For this review, take the finished solid that the model builds, in its own axes (mm). A direction names the side the tool comes from. Coordinates: 2 decimals unless noted, no trailing zeros. Loops run counter-clockwise (first coordinate to the right, second up) from the corner with the lowest first, then second, coordinate; pieces in that order, holes last. Notation, with made-up numbers: (-7, 27.25) -> (48, 27.25) arc R30 cw to (48, 58.25) -> close; hole circle Ø9 at (-33.75, -1). An arc over 180 degrees is marked (long way). One line per item, written item: value.
from build123d import *

# Parameters (mm, degrees)
IZIM1_W                                        = 46
IZIM1_H                                        = 22
Y_KSEKLIK_EKSTR_ZYON1_DEPTH                    = 35
IZIM2_W                                        = 40
IZIM2_H                                        = 22
KES_EKSTR_ZYON1_DEPTH                          = 32
RADYUS1_R                                      = 11
PAH1_SIZE                                      = 3
IZIM3_W                                        = 5
IZIM3_H                                        = 10
KES_EKSTR_ZYON2_DEPTH                          = 20
FEDER5_REACH                                   = 46.833
IZIM8_WALL_W                                   = 96.666047784
IZIM8_WALL_H                                   = 6
AYNALAMA4_COPY_1_REACH                         = 46.833
AYNALAMA4_COPY_1_SKETCH_W                      = 96.666047784
AYNALAMA4_COPY_1_SKETCH_H                      = 6
IZIM10_R                                       = 3.1
KES_EKSTR_ZYON4_DEPTH                          = 59.838762733
IZIM12_R                                       = 3.1
Y_KSEKLIK_EKSTR_ZYON3_DEPTH                    = 3
M3_D_Z_BA_L_MAKINE_VIDAS_IN_HAV_A1_D           = 2.5
M3_D_Z_BA_L_MAKINE_VIDAS_IN_HAV_A1_CSINK_D     = 3.1
M3_D_Z_BA_L_MAKINE_VIDAS_IN_HAV_A1_CSINK_ANGLE = 90
IZIM18_R                                       = 4
Y_KSEKLIK_EKSTR_ZYON4_DEPTH                    = 62.22
IZIM19_W                                       = 4
IZIM19_H                                       = 4
KES_EKSTR_ZYON5_DEPTH                          = 10
RADYUS2_R                                      = 1
Y_KSEKLIK_EKSTR_ZYON5_DEPTH                    = 2
Y_KSEKLIK_EKSTR_ZYON5_DEPTH_BACK               = 2
IZIM21_W                                       = 6
IZIM21_H                                       = 6
IZIM22_R                                       = 1.5
KES_EKSTR_ZYON6_DEPTH                          = 9
IZIM23_R                                       = 2.251355404
KES_EKSTR_ZYON7_DEPTH                          = 2
RADYUS3_R                                      = 1
M2_D_Z_BA_L_MAKINE_VIDAS_IN_HAV_A2_D           = 2
M2_D_Z_BA_L_MAKINE_VIDAS_IN_HAV_A2_DEPTH       = 46
M2_D_Z_BA_L_MAKINE_VIDAS_IN_HAV_A2_CSINK_D     = 4.4
M2_D_Z_BA_L_MAKINE_VIDAS_IN_HAV_A2_CSINK_ANGLE = 90
M2_D_Z_BA_L_MAKINE_VIDAS_IN_HAV_A2_TIP         = 0.600860619


# Read off the part's stored shape, not the designer's step: M2 Düz Başlı Makine Vidası İçin Havşa1
with BuildPart() as part:
    # Çizim1 → Yükseklik-Ekstrüzyon1 (new body)
    with BuildSketch(Plane(origin=(0, 0, 0), x_dir=(0, 0, -1), z_dir=(1, 0, 0))):
        Rectangle(IZIM1_W, IZIM1_H)
    extrude(amount=Y_KSEKLIK_EKSTR_ZYON1_DEPTH)

    # Çizim2 → Kes-Ekstrüzyon1 (cut)
    with BuildSketch(Plane(origin=(35, 0, 0), x_dir=(0, 0, -1), z_dir=(1, 0, 0))):
        Rectangle(IZIM2_W, IZIM2_H)
    extrude(amount=-KES_EKSTR_ZYON1_DEPTH, mode=Mode.SUBTRACT)

    # Radyus1
    radyus1_edges = [part.edges().sort_by_distance(p)[0] for p in [
        (35, -11, 21.5),
        (35, 11, 21.5),
        (35, -11, -21.5),
        (35, 11, -21.5),
    ]]
    fillet(radyus1_edges, radius=RADYUS1_R - 0.0001)  # a hair under: the kernel refuses the full size

    # Pah1
    pah1_edges = [part.edges().sort_by_distance(p)[0] for p in [
        (0, 0, 23),
        (0, 0, -23),
    ]]
    chamfer(pah1_edges, length=PAH1_SIZE)

    # Çizim3 → Kes-Ekstrüzyon2 (cut)
    with BuildSketch(Plane(origin=(-10, 0, 10), x_dir=(0.7071067811865468, 0, 0.7071067811865483), z_dir=(-0.7071067811865483, 0, 0.7071067811865468))):
        with Locations((16.262135624, 0)):
            Rectangle(IZIM3_W, IZIM3_H)
    kes_ekstr_zyon2 = extrude(amount=-KES_EKSTR_ZYON2_DEPTH, mode=Mode.SUBTRACT)

    # M2 Düz Başlı Makine Vidası İçin Havşa1 ou → M2 Düz Başlı Makine Vidası İçin Havşa1 (revolve, cut)
    with BuildSketch(Plane(origin=(24, -8, 0), x_dir=(1, 0, 0), z_dir=(0, -1, 0))):
        Polygon((0, 20), (1, 20), (1, 22.7), (1.3, 23), (0, 23), align=None)
    m2_d_z_ba_l_makine_vidas_in_hav_a1 = revolve(axis=Axis((24, -8, 0), (0, 0, 1)), mode=Mode.SUBTRACT)

    # M2 D_z Ba_l_ Makine Vidas_ _in Hav_a 2 → M2 D_z Ba_l_ Makine Vidas_ _in Hav_a1 2 (revolve, cut)
    with BuildSketch(Plane(origin=(32, 0, 0), x_dir=(1, 0, 0), z_dir=(0, -1, 0))):
        Polygon((0, 20), (1, 20), (1, 22.7), (1.3, 23), (0, 23), align=None)
    m2_d_z_ba_l_makine_vidas_in_hav_a1_2 = revolve(axis=Axis((32, 0, 0), (0, 0, 1)), mode=Mode.SUBTRACT)

    # M2 D_z Ba_l_ Makine Vidas_ _in Hav_a 3 → M2 D_z Ba_l_ Makine Vidas_ _in Hav_a1 3 (revolve, cut)
    with BuildSketch(Plane(origin=(24, 8, 0), x_dir=(1, 0, 0), z_dir=(0, -1, 0))):
        Polygon((0, 20), (1, 20), (1, 22.7), (1.3, 23), (0, 23), align=None)
    m2_d_z_ba_l_makine_vidas_in_hav_a1_3 = revolve(axis=Axis((24, 8, 0), (0, 0, 1)), mode=Mode.SUBTRACT)

    # M2 D_z Ba_l_ Makine Vidas_ _in Hav_a 4 → M2 D_z Ba_l_ Makine Vidas_ _in Hav_a1 4 (revolve, cut)
    with BuildSketch(Plane(origin=(16, 0, 0), x_dir=(1, 0, 0), z_dir=(0, -1, 0))):
        Polygon((0, 20), (1, 20), (1, 22.7), (1.3, 23), (0, 23), align=None)
    m2_d_z_ba_l_makine_vidas_in_hav_a1_4 = revolve(axis=Axis((16, 0, 0), (0, 0, 1)), mode=Mode.SUBTRACT)

    # Aynalama2: Kes-Ekstrüzyon2, M2 Düz Başlı Makine Vidası İçin Havşa1, M2 D_z Ba_l_ Makine Vidas_ _in Hav_a1 2, M2 D_z Ba_l_ Makine Vidas_ _in Hav_a1 3, M2 D_z Ba_l_ Makine Vidas_ _in Hav_a1 4 across plane
    add(kes_ekstr_zyon2.mirror(Plane.XY), mode=Mode.SUBTRACT)
    add(m2_d_z_ba_l_makine_vidas_in_hav_a1.mirror(Plane.XY), mode=Mode.SUBTRACT)
    add(m2_d_z_ba_l_makine_vidas_in_hav_a1_2.mirror(Plane.XY), mode=Mode.SUBTRACT)
    add(m2_d_z_ba_l_makine_vidas_in_hav_a1_3.mirror(Plane.XY), mode=Mode.SUBTRACT)
    add(m2_d_z_ba_l_makine_vidas_in_hav_a1_4.mirror(Plane.XY), mode=Mode.SUBTRACT)

    # Çizim8 wall → Feder5 (add, up to next)
    with BuildSketch(Plane(origin=(4.766833329, -5, -18.231299423), x_dir=(-0.706733233022, 0, 0.707480132118), z_dir=(0.707480132118, 0, 0.706733233022)), mode=Mode.PRIVATE) as feder5_sk1:
        with Locations((0, 3)):
            Rectangle(IZIM8_WALL_W, IZIM8_WALL_H)
    feder5_tool1 = extrude(feder5_sk1.sketch, amount=-FEDER5_REACH, mode=Mode.PRIVATE) - part.part
    feder5 = feder5_tool1.solids().sort_by_distance((4.766833329, -5, -18.231299423))[0]
    add(feder5)

    # Aynalama3: Feder5 across plane
    add(feder5.mirror(Plane.ZX))

    # Aynalama4: Feder5 across plane
    add(feder5.mirror(Plane.XY))

    # Aynalama4 copy 1 sketch → Aynalama4 copy 1 (add, up to next)
    with BuildSketch(Plane(origin=(4.766833329, 5, 18.231299423), x_dir=(-0.706733233022, 0, -0.707480132118), z_dir=(0.707480132118, 0, -0.706733233022)), mode=Mode.PRIVATE) as aynalama4_copy_1_sk1:
        with Locations((0, 3)):
            Rectangle(AYNALAMA4_COPY_1_SKETCH_W, AYNALAMA4_COPY_1_SKETCH_H)
    aynalama4_copy_1_tool1 = extrude(aynalama4_copy_1_sk1.sketch, amount=-AYNALAMA4_COPY_1_REACH, mode=Mode.PRIVATE) - part.part
    add(aynalama4_copy_1_tool1.solids().sort_by_distance((4.766833329, 5, 18.231299423))[0])

    # Çizim10 → Kes-Ekstrüzyon4 (cut, through all)
    with BuildSketch(Plane(origin=(0, 0, -23), x_dir=(-1, 0, 0), z_dir=(0, 0, -1))):
        with Locations(Location((-24, 0, 0), (0, 0, 90))):
            Circle(IZIM10_R)
    extrude(amount=-KES_EKSTR_ZYON4_DEPTH, mode=Mode.SUBTRACT)

    # Çizim12 → Yükseklik-Ekstrüzyon3 (add)
    with BuildSketch(Plane(origin=(0, 0, -23), x_dir=(-1, 0, 0), z_dir=(0, 0, -1))):
        with Locations(Location((-24, 0, 0), (0, 0, 90))):
            Circle(IZIM12_R)
    extrude(amount=-Y_KSEKLIK_EKSTR_ZYON3_DEPTH)

    # M3 Düz Başlı Makine Vidası İçin Havşa1 (through all)
    with Locations(Plane(origin=(24, 0, -23), x_dir=(0, -1, 0), z_dir=(0, 0, -1))):
        with Locations((0, 0)):
            CounterSinkHole(M3_D_Z_BA_L_MAKINE_VIDAS_IN_HAV_A1_D / 2, M3_D_Z_BA_L_MAKINE_VIDAS_IN_HAV_A1_CSINK_D / 2, counter_sink_angle=M3_D_Z_BA_L_MAKINE_VIDAS_IN_HAV_A1_CSINK_ANGLE)

    # Çizim18 → Yükseklik-Ekstrüzyon4 (add)
    with BuildSketch(Plane.ZY):
        with Locations(Location((0, 0, 0), (0, 0, 180))):
            Circle(IZIM18_R)
    extrude(amount=Y_KSEKLIK_EKSTR_ZYON4_DEPTH)

    # Çizim19 → Kes-Ekstrüzyon5 (cut)
    with BuildSketch(Plane.ZY.offset(62.22)):
        Rectangle(IZIM19_W, IZIM19_H)
    extrude(amount=-KES_EKSTR_ZYON5_DEPTH, mode=Mode.SUBTRACT)

    # Çizim20 → Döndür1 (revolve)
    with BuildSketch(Plane.XY, mode=Mode.PRIVATE) as d_nd_r1_sk:
        Polygon((-52.22, -1.75), (-52.22, -3.5), (-53.97, -3.5), align=None)
    revolve(d_nd_r1_sk.sketch.rotate(Axis((-62.22, 0, 0), (1, 0, 0)), 270), axis=Axis((-62.22, 0, 0), (1, 0, 0)))

    # Radyus2
    radyus2_edges = [part.edges().sort_by_distance(p)[0] for p in [
        (0, 0, 4),
    ]]
    fillet(radyus2_edges, radius=RADYUS2_R)

    # Çizim21 → Yükseklik-Ekstrüzyon5 (add, two sides: drawn at the far end of the back side and taken through both)
    with BuildSketch(Plane(origin=(0, 4, 0), x_dir=(1, 0, 0), z_dir=(0, 1, 0)).offset(-Y_KSEKLIK_EKSTR_ZYON5_DEPTH_BACK)):
        with Locations((-55.22, 0)):
            Rectangle(IZIM21_W, IZIM21_H)
    extrude(amount=Y_KSEKLIK_EKSTR_ZYON5_DEPTH + Y_KSEKLIK_EKSTR_ZYON5_DEPTH_BACK)

    # Çizim22 → Kes-Ekstrüzyon6 (cut)
    with BuildSketch(Plane(origin=(0, 6, 0), x_dir=(1, 0, 0), z_dir=(0, 1, 0))):
        with Locations(Location((-55.22, 0, 0), (0, 0, 270))):
            Circle(IZIM22_R)
    extrude(amount=-KES_EKSTR_ZYON6_DEPTH, mode=Mode.SUBTRACT)

    # Çizim23 → Kes-Ekstrüzyon7 (cut)
    with BuildSketch(Plane(origin=(0, 6, 0), x_dir=(1, 0, 0), z_dir=(0, 1, 0))):
        with Locations(Location((-55.22, 0, 0), (0, 0, 270))):
            Circle(IZIM23_R)
    extrude(amount=-KES_EKSTR_ZYON7_DEPTH, mode=Mode.SUBTRACT)

    # Radyus3
    radyus3_edges = [part.edges().sort_by_distance(p)[0] for p in [
        (-55.22, 2.645751311, 3),
        (-55.22, 2.645751311, -3),
        (-52.22, 4, 0),
        (-58.22, 4, 0),
    ]]
    fillet(radyus3_edges, radius=RADYUS3_R)

    # M2 Düz Başlı Makine Vidası İçin Havşa2
    with Locations(Plane.XZ.offset(4)):
        with Locations((-55.22, 0)):
            CounterSinkHole(M2_D_Z_BA_L_MAKINE_VIDAS_IN_HAV_A2_D / 2, M2_D_Z_BA_L_MAKINE_VIDAS_IN_HAV_A2_CSINK_D / 2, depth=M2_D_Z_BA_L_MAKINE_VIDAS_IN_HAV_A2_DEPTH, counter_sink_angle=M2_D_Z_BA_L_MAKINE_VIDAS_IN_HAV_A2_CSINK_ANGLE)
            with Locations((0, 0, -(M2_D_Z_BA_L_MAKINE_VIDAS_IN_HAV_A2_DEPTH + M2_D_Z_BA_L_MAKINE_VIDAS_IN_HAV_A2_TIP / 2))):  # 118° drill point
                Cone(0, M2_D_Z_BA_L_MAKINE_VIDAS_IN_HAV_A2_D / 2, M2_D_Z_BA_L_MAKINE_VIDAS_IN_HAV_A2_TIP, mode=Mode.SUBTRACT)


solid = part.part
1. To check wall thickness, follow probe 1 along Y at (x, z) = (24, -22); probe 2 along X at (y, z) = (2.5, 0); probe 3 along Z at (x, y) = (15.5, -2.5). State the ranges of each line that lie inside material, in increasing order. Write a range as from..to.
Return value:
probe 1: y = -11..-9, -7..-1.25, 1.25..7, 9..11
probe 2: x = -62.22..-56.72, -53.72..3
probe 3: z = -23..-20, 20..23
2. Insertion check: pin 1 Ø8 at (x, y) = (-29.5, 5) entering from +Z; pin 2 Ø2.5 at (x, z) = (-55.22, 0) entering from +Y; pin 3 Ø2.5 at (x, y) = (16, 0) entering from +Z. Each pin has a flat end and moves straight along its axis. Give the tip position at first contact, or say it passes through.
Return value:
pin 1: stops at z = 3.87
pin 2: stops at y = -3
pin 3: stops at z = 22.95
3. For faces 4 (the flat face through (-57, 4, 0)), 5 (the flat face through (-58, 2, 0)), 6 (the flat face through (-55, 4, 3)), 7 (the flat face through (21, 0, -20)), list the 3-axis set-ups (+Z, -Z, +X, -X, +Y, -Y) from which the entire face can be reached by the end or side of a thin tool; tool diameter is ignored.
Return value:
face 4: +Y
face 5: -X
face 6: +Z, -X, +Y
face 7: +X, +Y, -Y
4. The part is to be moulded in two halves that separate along Y. For faces 1 (the flat face through (18, 0, 20)), 2 (the flat face through (2, -11, 1)), 3 (the flat face through (3, 5, 20)), say which applies: pulls with the +Y half, pulls with the -Y half, needs draft (parallel to the pull), parting line crosses it, or undercut.
Return value:
face 1: needs draft
face 2: pulls with the -Y half
face 3: undercut
5. Take a section at C-C, the plane z = 0. Give the number of separate pieces and of enclosed holes in the cut face, and give its area (3 significant figures).
Return value:
separate pieces: 3
enclosed holes: 0
area: 515 mm2
6. Take a section at B-B, the plane y = 8. Give the boundary of the cut face in (x, z), and give its area (3 significant figures).
Return value:
outline: (0, -20) -> (3, -23) -> (22.7, -23) -> (23, -22.7) -> (23, -20) -> (6.53, -20) -> (3, -16.46) -> (3, 16.46) -> (6.53, 20) -> (23, 20) -> (23, 22.7) -> (22.7, 23) -> (3, 23) -> (0, 20) -> close; (25, -22.7) -> (25.3, -23) -> (31.55, -23) -> (31.55, -20) -> (25, -20) -> close; (25, 20) -> (31.55, 20) -> (31.55, 23) -> (25.3, 23) -> (25, 22.7) -> close
area: 301 mm2
7. Take a section at D-D, the plane x = -55.22. Give the boundary of the cut face in (y, z), and give its area (3 significant figures).
Return value:
outline: (-3.58, -1.78) arc R4 ccw to (2.4, -3.2) arc R1 cw to (3, -3) -> (6, -3) -> (6, -2.25) -> (4, -2.25) -> (4, -1.5) -> (2, -1.5) -> (2, -2) -> (-2, -2) -> (-2, -1.5) -> (-3, -1.5) -> (-3, -1.2) -> close; (-3.58, 1.78) -> (-3, 1.2) -> (-3, 1.5) -> (-2, 1.5) -> (-2, 2) -> (2, 2) -> (2, 1.5) -> (4, 1.5) -> (4, 2.25) -> (6, 2.25) -> (6, 3) -> (3, 3) arc R1 cw to (2.4, 3.2) arc R4 ccw to start
area: 28.0 mm2
8. Take a section at A-A, the plane x = 16. Give the boundary of the cut face in (y, z), and give its area (3 significant figures).
Return value:
outline: (-11, -23) -> (-1.3, -23) -> (-1, -22.7) -> (-1, -20) -> (-11, -20) -> close; (-11, 20) -> (-1, 20) -> (-1, 22.7) -> (-1.3, 23) -> (-11, 23) -> close; (1, -22.7) -> (1.3, -23) -> (11, -23) -> (11, -20) -> (1, -20) -> close; (1, 20) -> (11, 20) -> (11, 23) -> (1.3, 23) -> (1, 22.7) -> close
area: 120 mm2
